Input: part model. Units: mm. Frame: model coordinates. A direction names the side the tool comes from. Coordinates: 2 decimals unless noted, no trailing zeros. Write each loop counter-clockwise with the first axis right and the second up, starting at its lowest first coordinate (ties: lowest second). Pieces come first, ordered by that corner, then holes. Notation, with made-up numbers: M 29.5,-38.5 L 43.5,-38.5 A16 ccw 43.5,-26.5 Z; hole C -31,27.5 d10. An arc over 180 degrees is marked long. Use CSV: the item, a comma, the result in double quotes.
```python
from build123d import *

# Parameters (mm, degrees)
F0_R     = 4.191
F1_DEPTH = 10
F2_R     = 1.651
F3_DEPTH = 5
F6_DEPTH = 2


with BuildPart() as f1:
    # F0 (on Top) → F1 (new body)
    with BuildSketch(Plane.XY):
        Circle(F0_R)
    extrude(amount=F1_DEPTH)

    # F2 (on Top) → F3 (cut)
    with BuildSketch(Plane.XY):
        Circle(F2_R)
    extrude(amount=F3_DEPTH, mode=Mode.SUBTRACT)

    # F5 (on offset) → F6 (join)
    with BuildSketch(Plane.XZ.offset(1)):
        with BuildLine():
            Line((-16.51, 1.89748), (-8.89, 1.89748))
            Line((-8.89, 1.89748), (-8.89, 5.08))
            Line((-8.89, 5.08), (-8.89, 12.05748))
            Line((-8.89, 12.05748), (-16.51, 12.05748))
            ThreePointArc((-16.51, 12.05748), (-18.306051, 11.313531), (-19.05, 9.51748))
            Line((-19.05, 9.51748), (-19.05, 4.43748))
            ThreePointArc((-19.05, 4.43748), (-18.306051, 2.641429), (-16.51, 1.89748))
        make_face()
        Polygon((-8.89, 1.89748), (-3.046233, 3.931247), (-3.046233, 10.023713), (-8.89, 12.05748), (-8.89, 5.08), align=None)
        Polygon((3.046233, 3.931247), (8.89, 1.89748), (8.89, 5.08), (8.89, 12.05748), (3.046233, 10.023713), align=None)
        with BuildLine():
            Line((8.89, 5.08), (8.89, 1.89748))
            Line((8.89, 1.89748), (16.51, 1.89748))
            ThreePointArc((16.51, 1.89748), (18.306051, 2.641429), (19.05, 4.43748))
            Line((19.05, 4.43748), (19.05, 9.51748))
            ThreePointArc((19.05, 9.51748), (18.306051, 11.313531), (16.51, 12.05748))
            Line((16.51, 12.05748), (8.89, 12.05748))
            Line((8.89, 12.05748), (8.89, 5.08))
        make_face()
    extrude(amount=-F6_DEPTH)


solid = f1.part
```
1. Contact query for flat-ended pins moving along their axis: pin 1 Ø5 at (x, z) = (-11.5, 9) entering from +Y; pin 2 Ø0.6 at (x, y) = (11, 0) entering from -Z; pin 3 Ø4 at (x, z) = (-9.5, 2) entering from -Y. Output: stop coordinate, or through.
Resolved:
pin 1,"stops at y = 1"
pin 2,"stops at z = 1.9"
pin 3,"stops at y = -1"
2. Section A-A (x = 0). Return loops of the section in (y, z).
Resolved:
outline,"M -4.19,0 L -1.65,0 L -1.65,5 L 1.65,5 L 1.65,0 L 4.19,0 L 4.19,10 L -4.19,10 Z"
3. Access query for faces 1 (the flat face through (0, 0, 5)), 2 (the flat face through (13, 0, 1.897)), 3 (the flat face through (-13, 0, 1.897)), 4 (the flat face through (-5.927, -0.014, 11.026)), 5 (the flat face through (13, 1, 7)). Directions: +Z, -Z, +X, -X, +Y, -Y. A direction counts if a zero-diameter tool reaches every point of the face in a straight line with its end or side. Return the directions, or none.
Resolved:
face 1,"-Z"
face 2,"-Z, +X, +Y, -Y"
face 3,"-Z, -X, +Y, -Y"
face 4,"+Z, +Y, -Y"
face 5,"+Z, -Z, +X, +Y"
4. Section D-D (z = 10.5). Return loops of the section in (x, y), then the cut area to 4 significant figures.
Resolved:
outline,"M -18.85,-1 L -4.41,-1 L -4.41,1 L -18.85,1 Z; M 4.41,-1 L 18.85,-1 L 18.85,1 L 4.41,1 Z"
area,"57.75 mm^2"
5. Section B-B (z = 9). Return loops of the section in (x, y).
Resolved:
outline,"M -19.05,-1 L -4.07,-1 A4.19 ccw 4.07,-1 L 19.05,-1 L 19.05,1 L 4.07,1 A4.19 ccw -4.07,1 L -19.05,1 Z"
6. Material intervals for line 1 (Y direction, x = 0, z = 3.7); line 2 (Y direction, x = -17, z = 4.5); line 3 (Z direction, x = -15.5, y = 0.25), sorted ascending. Write a range as [from, to].
Resolved:
line 1,"y = [-4.19, -1.65], [1.65, 4.19]"
line 2,"y = [-1, 1]"
line 3,"z = [1.9, 12.06]"
7. Mould query, pull axis X, two halves, no side actions, for faces 6 (the cylindrical face through (-18.29, -0.01, 11.33)), 7 (the flat face through (6.009, -0.014, 11.055)), 8 (the cylindrical face through (18.33, -0.01, 11.29)). Classes: pulls with the +X half, pulls with the -X half, needs draft (parallel to the pull), parting line crosses it, or undercut.
Resolved:
face 6,"pulls with the -X half"
face 7,"undercut"
face 8,"pulls with the +X half"
